```python
from build123d import *

# Parameters (mm, degrees)
BOSS_EXTRUDE1_DEPTH = 3
CUT_EXTRUDE1_DEPTH  = 10


with BuildPart() as part:
    # Sketch1 → Boss-Extrude1 (new body)
    with BuildSketch(Plane.XY):
        with BuildLine():
            add(Edge.make_bspline(
                [(-70, -11.5), (-70, 26.5), (-18, 33.5), (-10, 33.5)],
                knots=[0, 0, 0, 0, 1, 1, 1, 1], degree=3))
            Line((-70, -11.5), (-70, -46.5))
            ThreePointArc((-70, -46.5), (-55.355339059, -81.855339059), (-20, -96.5))
            Line((-20, -96.5), (20, -96.5))
            ThreePointArc((20, -96.5), (55.355339059, -81.855339059), (70, -46.5))
            Line((70, -46.5), (70, -11.5))
            add(Edge.make_bspline(
                [(10, 33.5), (18, 33.5), (70, 26.5), (70, -11.5)],
                knots=[0, 0, 0, 0, 1, 1, 1, 1], degree=3))
            Line((10, 33.5), (-10, 33.5))
        make_face()
    extrude(amount=BOSS_EXTRUDE1_DEPTH)

    # Sketch2 → Cut-Extrude1 (cut)
    with BuildSketch(Plane.XY.offset(3)):
        with BuildLine():
            Line((-22.5, -40), (22.5, -40))
            ThreePointArc((22.5, -40), (29.571067812, -37.071067812), (32.5, -30))
            Line((32.5, -30), (32.5, 5))
            ThreePointArc((32.5, 5), (29.571067812, 12.071067812), (22.5, 15))
            Line((22.5, 15), (-22.5, 15))
            ThreePointArc((-22.5, 15), (-29.571067812, 12.071067812), (-32.5, 5))
            Line((-32.5, 5), (-32.5, -30))
            ThreePointArc((-32.5, -30), (-29.571067812, -37.071067812), (-22.5, -40))
        make_face()
    extrude(amount=-CUT_EXTRUDE1_DEPTH, mode=Mode.SUBTRACT)


solid = part.part
```
Work out the finished part from the listing and answer in its coordinate system (mm). A direction names the side the tool comes from. Give positions to 0.01 mm unless a question says otherwise; leave off trailing zeros. Loops run counter-clockwise (first coordinate to the right, second up) from the corner with the lowest first, then second, coordinate; pieces in that order, holes last. Notation, with made-up numbers: (82.25, 55.25) -> (141.25, 55.25) arc R19 cw to (141.25, 70.25) -> close; hole circle Ø10 at (84.25, 10). An arc over 180 degrees is marked (long way). Put each result on its own line as item: value. Start each with the question number.
Item 1: The part is cut by section C-C (y = -67). Give the vertices of the cut face in (x, z), then the cut area to 3 significant figures.
Item 2: Find the intervals of material crossed by L1, parallel to X at y = -13.5, z = 2.6; L2, parallel to Y at x = 8, z = 2.8; L3, parallel to X at y = -47.5, z = 1.9, in increasing order. Write a range as [from, to].
Item 3: The mould has two halves that part along X. Classify faces 3 (the face through (1, -45, 3)), 4 (the face through (0, 15, 2)), 5 (the face through (-70, -29, 1)): released by +X, released by -X, zero draft, split by the parting line, or undercut.
Item 4: The part is cut by section B-B (y = -26). Give the vertices of the cut face in (x, z), then the cut area to 3 significant figures.
Item 5: Which of the six approach directions +Z, -Z, +X, -X, +Y, -Y give full straight-line access (tool end or side, diameter ignored) to faces 1 (the face through (1, -45, 0)), 2 (the face through (0, -40, 2))?
Item 6: This flat-tipped pin is pushed along its axis until it touches: P1, Ø1.5, axis at x = 29, z = 0.5, coming from the -Y side. Where does it stop, or does it pass through?
Item 7: The part is cut by section A-A (x = 6.5). Give the vertices of the cut face in (y, z).
Answers below:
1. outline: (-65.6, 0) -> (65.6, 0) -> (65.6, 3) -> (-65.6, 3) -> close
1. area: 394 mm2
2. L1: [-70, -32.5], [32.5, 70]
2. L2: [-96.5, -40], [15, 33.5]
2. L3: [-69.99, 69.99]
3. face 3: zero draft
3. face 4: undercut
3. face 5: released by -X
4. outline: (-70, 0) -> (-32.5, 0) -> (-32.5, 3) -> (-70, 3) -> close; (32.5, 0) -> (70, 0) -> (70, 3) -> (32.5, 3) -> close
4. area: 225 mm2
5. face 1: -Z, +X, -X, +Y, -Y
5. face 2: +Z, -Z
6. P1: y = -95.81
7. outline: (-96.5, 0) -> (-40, 0) -> (-40, 3) -> (-96.5, 3) -> close; (15, 0) -> (33.5, 0) -> (33.5, 3) -> (15, 3) -> close
